For this review, take the finished solid that the model builds, in its own axes (mm). A direction names the side the tool comes from. Round coordinates to 2 decimals unless told otherwise and drop trailing zeros. Use a Markdown table: item, result.
from build123d import *

# Parameters (mm, degrees)
SKETCH1_R           = 2.1
BOSS_EXTRUDE2_DEPTH = 495.3


with BuildPart() as part:
    # Sketch1 → Boss-Extrude2 (new body)
    with BuildSketch(Plane(origin=(0, 0, 0), x_dir=(0, 0, -1), z_dir=(1, 0, 0))):
        Polygon((-20, -4.6), (-20, -10), (-14.6, -10), (-13.1, -8.5), (-15.5, -8.5), (-15.5, -7), (-13.1, -4.5), (-6.9, -4.5), (-4.5, -7), (-4.5, -8.5), (-6.9, -8.5), (-5.4, -10), (0, -10), (0, -8.5), (-3, -8.5), (-3, -6.396534569), (-5.5, -3.792367902), (-5.5, 3.792367902), (-3, 6.396534569), (-3, 8.5), (0, 8.5), (0, 10), (-5.4, 10), (-6.9, 8.5), (-4.5, 8.5), (-4.5, 7), (-6.9, 4.5), (-13.1, 4.5), (-15.5, 7), (-15.5, 8.5), (-13.1, 8.5), (-14.6, 10), (-20, 10), (-20, 4.6), (-18.5, 3.1), (-18.5, 6.396534569), (-17, 6.396534569), (-14.5, 3.792367902), (-14.5, -3.792367902), (-17, -6.396534569), (-18.5, -6.396534569), (-18.5, -3.1), align=None)
        with Locations((-10, 0)):
            Circle(SKETCH1_R, mode=Mode.SUBTRACT)
        Polygon((0, -8.5), (0, -10), (5.4, -10), (6.9, -8.5), (4.5, -8.5), (4.5, -7), (6.9, -4.5), (13.1, -4.5), (15.5, -7), (15.5, -8.5), (13.1, -8.5), (14.6, -10), (20, -10), (20, -4.6), (18.5, -3.1), (18.5, -6.396534569), (17, -6.396534569), (14.5, -3.792367902), (14.5, 3.792367902), (17, 6.396534569), (18.5, 6.396534569), (18.5, 3.1), (20, 4.6), (20, 10), (14.6, 10), (13.1, 8.5), (15.5, 8.5), (15.5, 7), (13.1, 4.5), (6.9, 4.5), (4.5, 7), (4.5, 8.5), (6.9, 8.5), (5.4, 10), (0, 10), (0, 8.5), (3, 8.5), (3, 6.396534569), (5.5, 3.792367902), (5.5, -3.792367902), (3, -6.396534569), (3, -8.5), align=None)
        with Locations((10, 0)):
            Circle(SKETCH1_R, mode=Mode.SUBTRACT)
    extrude(amount=BOSS_EXTRUDE2_DEPTH)


solid = part.part
Q1. Wall thickness on line 1 along Y through (x, z) = (130.5, -10); line 2 along Z through (x, y) = (175.5, 3.25); line 3 along Z through (x, y) = (124, -6.5): over which ranges is each line inside the solid? List them lowest first. Write a range as [from, to].
Determined:
| item | result |
|---|---|
| line 1 | y = [-4.5, -2.1], [2.1, 4.5] |
| line 2 | z = [-18.65, -18.5], [-14.5, -5.5], [5.5, 14.5], [18.5, 18.65] |
| line 3 | z = [-20, -15.02], [-4.98, -3], [3, 4.98], [15.02, 20] |
Q2. Machinability: for faces 1 (the flat face through (495.3, -6.5, 4.7)), 2 (the flat face through (244, 0, -14.5)), which of the approach directions +Z, -Z, +X, -X, +Y, -Y give a long, thin tool a straight path to every point of the face, cutting with its end or side? Answer none if there is none.
Determined:
| item | result |
|---|---|
| face 1 | +Z, -Z, +X, +Y, -Y |
| face 2 | +X, -X |
Q3. Draft analysis for pull direction Z (two halves, no side actions). For faces 3 (the flat face through (244, -10, 0)), 4 (the flat face through (244, 0, -5.5)), state which applies: pulls with the +Z half, pulls with the -Z half, needs draft (parallel to the pull), parting line crosses it, or undercut.
Determined:
| item | result |
|---|---|
| face 3 | needs draft |
| face 4 | undercut |
Q4. Add section A-A (x = 86.5). Give the number of separate pieces and of enclosed holes in the cut face, then the cut area to 3 significant figures.
Determined:
| item | result |
|---|---|
| separate pieces | 1 |
| enclosed holes | 3 |
| area | 309 mm^2 |
Q5. Clearance check with flat-ended pins moving along their axes: pin 1 (3 mm diameter, centred on x = 199.5, z = -10.5, fed in from -Y); pin 2 (6 mm diameter, centred on x = 238, y = 1.5, fed in from +Z); pin 3 (1.5 mm diameter, centred on x = 323, z = 7.5, fed in from +Y). State where each tip first meets the part, or that it passes through.
Determined:
| item | result |
|---|---|
| pin 1 | stops at y = -4.5 |
| pin 2 | stops at z = 19.9 |
| pin 3 | stops at y = 8.65 |
